Check sheet for the drawn part. Datum: minimum x, y, z corner. Units: mm. A direction names the side the tool comes from. Give positions to 0.01 mm unless a question says otherwise; leave off trailing zeros. Loops run counter-clockwise (first coordinate to the right, second up) from the corner with the lowest first, then second, coordinate; pieces in that order, holes last.
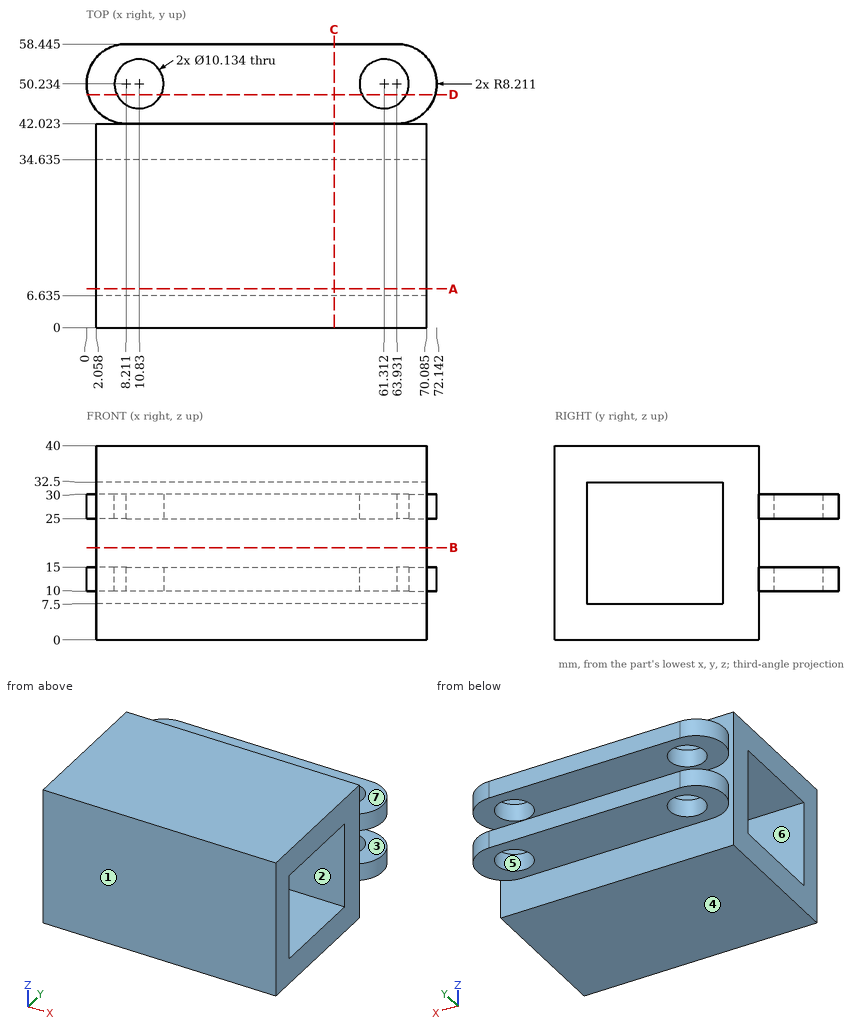
1) Sectioned sample at B-B on z = 19. Enter the section's corners in (x, y) (1 decimal).
2) Mould release check, pull along Z, two halves, no side actions. Record for the marked faces 4, 5, 6 and 7: +Z half, -Z half, draft (parallel to the pull), parting line (faces both ways), or undercut.
3) Depth check by flat-ended pin: P1, Ø12, axis at y = 15, z = 24, coming from the -X side; P2, Ø2, axis at x = 47, z = 8, coming from the +Y side; P3, Ø16, axis at x = 10.83, y = 50.23, coming from the -Z side; P4, Ø8, axis at x = 30, y = 51, coming from the +Z side. Enter the tip coordinate at first touch or a pass-through.
4) Sectioned sample at A-A on y = 8. Enter the section's corners in (x, z) (1 decimal), plus the area to 3 significant figures.
5) Scan lines: line 1 along Y through (x, z) = (61.5, 10.5) (1 decimal); line 2 along Y through (x, z) = (13.5, 22.5) (1 decimal); line 3 along Z through (x, y) = (54.5, 32.5). Record each from-to range of solid material in increasing order.
6) Sectioned sample at C-C on x = 51. Enter the section's corners in (y, z) (1 decimal), plus the area to 4 significant figures.
7) Sectioned sample at D-D on y = 48. Enter the section's corners in (x, z) (1 decimal).
8) Tool access check on the marked faces 1, 2 and 3. Record the directions out of +Z, -Z, +X, -X, +Y, -Y that give a thin tool (end or side, any length) a straight path to the whole face; none if there is none.
Determined:
1. outline: (2.1, 0) - (70.1, 0) - (70.1, 6.6) - (2.1, 6.6) - close; (2.1, 34.6) - (70.1, 34.6) - (70.1, 42) - (2.1, 42) - close
2. face 4: -Z half
2. face 5: draft
2. face 6: undercut
2. face 7: +Z half
3. P1: passes through
3. P2: stops at y = 42.02
3. P3: stops at z = 10
3. P4: stops at z = 30
4. outline: (2.1, 0) - (70.1, 0) - (70.1, 7.5) - (2.1, 7.5) - close; (2.1, 32.5) - (70.1, 32.5) - (70.1, 40) - (2.1, 40) - close
4. area: 1,020 mm2
5. line 1: y = 0 to 6.6, 34.6 to 45.2, 55.3 to 58.4
5. line 2: y = 0 to 6.6, 34.6 to 42
5. line 3: z = 0 to 7.5, 32.5 to 40
6. outline: (0, 0) - (42, 0) - (42, 10) - (58.4, 10) - (58.4, 15) - (42, 15) - (42, 25) - (58.4, 25) - (58.4, 30) - (42, 30) - (42, 40) - (0, 40) - close; hole (6.6, 7.5) - (34.6, 7.5) - (34.6, 32.5) - (6.6, 32.5) - close
6. area: 1,145 mm2
7. outline: (0.3, 10) - (6.3, 10) - (6.3, 15) - (0.3, 15) - close; (0.3, 25) - (6.3, 25) - (6.3, 30) - (0.3, 30) - close; (15.4, 10) - (56.8, 10) - (56.8, 15) - (15.4, 15) - close; (15.4, 25) - (56.8, 25) - (56.8, 30) - (15.4, 30) - close; (65.9, 10) - (71.8, 10) - (71.8, 15) - (65.9, 15) - close; (65.9, 25) - (71.8, 25) - (71.8, 30) - (65.9, 30) - close
8. face 1: +Z, -Z, +X, -X, -Y
8. face 2: +X, -X
8. face 3: +X, -X, +Y
